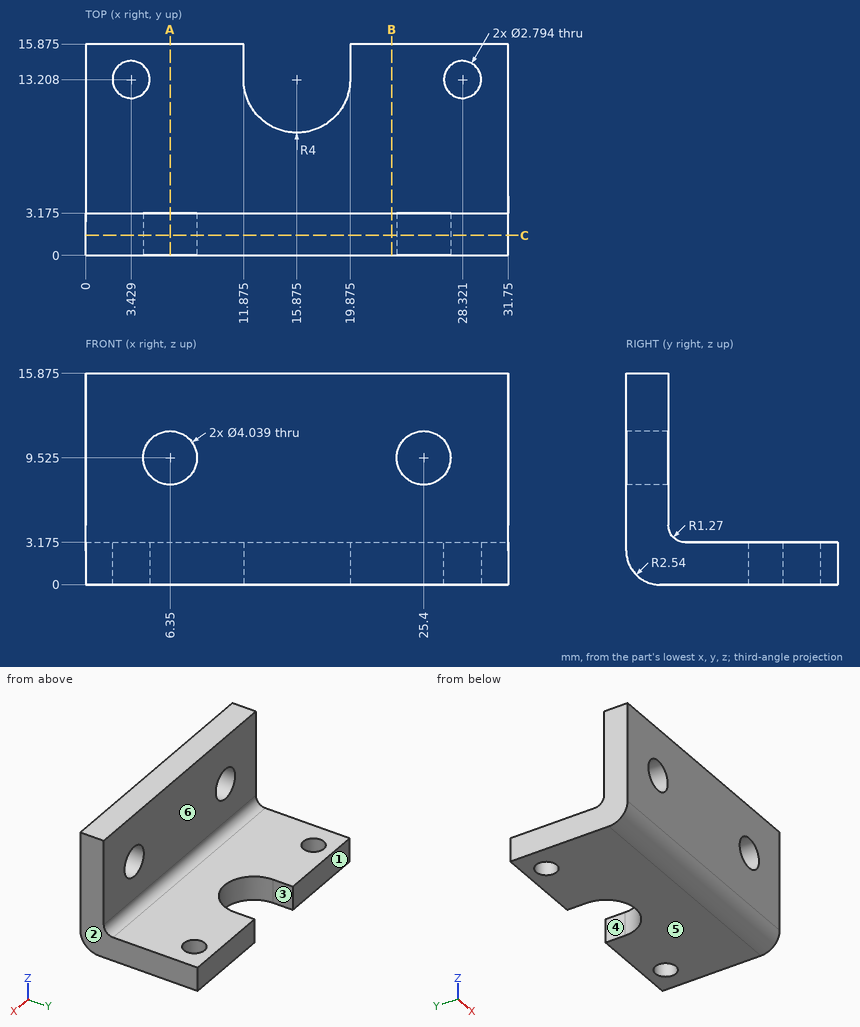
Can you work these out from the drawing? Everything is in mm from the part's minimum corner. A direction names the side the tool comes from. Coordinates: 2 decimals unless noted, no trailing zeros. Loops run counter-clockwise (first coordinate to the right, second up) from the corner with the lowest first, then second, coordinate; pieces in that order, holes last. Notation, with made-up numbers: M 21.5,87.5 L 56.5,87.5 A16 cw 56.5,110.5 Z; hole C -0.5,67 d7. An arc over 180 degrees is marked long. Put each result on its own line as item: value. Start each with the question number.
(1) Suppose I cut it at B-B on x = 23. Please give me the cut outline in (y, z) (1 decimal).
(2) Thinking about a two-plate mould opening in X: for the marked faces 1, 2 and 3, which applies, pulls with the +X half, pulls with the -X half, needs draft (parallel to the pull), parting line crosses it, or undercut?
(3) I need wall thicknesses on line 1 (X direction, y = 0.5, z = 11); line 2 (Z direction, x = 13.5, y = 6) (1 decimal). Which ranges of each line are inside material? Lowest first, please. Write a range as from..to.
(4) Suppose I cut it at A-A on x = 6.35. Please give me the cut outline in (y, z) (1 decimal).
(5) For the marked faces 4, 5 and 6, which set-ups out of +Z, -Z, +X, -X, +Y, -Y let a thin tool reach every point of the face, with its end or its side?
(6) Suppose I cut it at C-C on y = 1.5. Count the separate pieces of the cut face and the enclosed holes in it, then the cut area to 3 significant figures.
(7) Will these pins go through, and if not, where does the flat tip stop? P1, Ø8, axis at x = 11, y = 13.5, coming from the +Z side (1 decimal); P2, Ø4, axis at x = 13, z = 13.5, coming from the +Y side (1 decimal).
Solutions:
1. outline: M 0,2.5 A2.5 ccw 2.5,0 L 15.9,0 L 15.9,3.2 L 4.4,3.2 A1.3 cw 3.2,4.4 L 3.2,15.9 L 0,15.9 Z
2. face 1: needs draft
2. face 2: pulls with the +X half
2. face 3: undercut
3. line 1: x = 0..4.97, 7.73..24.02, 26.78..31.75
3. line 2: z = 0..3.2
4. outline: M 0,2.5 A2.5 ccw 2.5,0 L 15.9,0 L 15.9,3.2 L 4.4,3.2 A1.3 cw 3.2,4.4 L 3.2,7.5 L 0,7.5 Z; M 0,11.5 L 3.2,11.5 L 3.2,15.9 L 0,15.9 Z
5. face 4: +Z, -Z, +Y
5. face 5: -Z, +X, -X, +Y, -Y
5. face 6: +Z, +X, -X, +Y
6. separate pieces: 1
6. enclosed holes: 2
6. area: 471 mm2
7. P1: stops at z = 3.2
7. P2: stops at y = 3.2
